Verification items for the finished model (mm, model axes). Face numbers are marked on the shaded views. Give positions to 0.01 mm unless a question says otherwise; leave off trailing zeros. Order: outer loops, then holes, each group sorted by start corner. A loop starts at its lowest first (then second) coordinate and runs counter-clockwise, first axis right, second up.
(1) Sectioned sample at D-D on z = 15. Record the cut outline in (x, y).
(2) Scan lines: L1, parallel to Z at x = 0, y = 0.45; L2, parallel to Z at x = 0, y = 2.15; L3, parallel to Y at x = -25, z = -4.5. Record each from-to range of solid material in increasing order.
(3) Sectioned sample at B-B on z = 0. Record the cut outline in (x, y), plus the area to 3 significant figures.
(4) Sectioned sample at A-A on x = 0. Record the cut outline in (y, z).
(5) Mould release check, pull along Z, two halves, no side actions. Record for the marked faces 1, 2 and 3: pulls with the +Z half, pulls with the -Z half, needs draft (parallel to the pull), parting line crosses it, or undercut.
(6) Sectioned sample at C-C on y = 19. Record the cut outline in (x, z).
(7) Gauge pin test, flat ends, axial feed: pin 1 (10 mm diameter, centred on y = 16, z = 23.5, fed in from +X); pin 2 (4 mm diameter, centred on y = 19, z = 13.5, fed in from -X); pin 3 (1 mm diameter, centred on y = 4.5, z = 27.5, fed in from -X). Record the tip position at first contact, or that the pin passes through.
Autodesk Inventor part; units mm, degrees
ref_plane "YZ Plane" through (0, 0, 0) normal (1, 0, 0) x (0, 1, 0)
ref_plane "XZ Plane" through (0, 0, 0) normal (0, 1, 0) x (-1, 0, 0)
ref_plane "XY Plane" through (0, 0, 0) normal (0, 0, 1) x (1, 0, 0)
sketch "Sketch1" plane through (0, 0, 0) normal (0, 1, 0) x (-1, 0, 0)
  circle A0 centre (0, 0) radius 44
  dimension "d0" = 88
extrude "Extrusion1" add sketch "Sketch1" along normal blind 25
sketch "Sketch2" plane through (0, 25, 0) normal (0, 1, 0) x (1, 0, 0)
  circle A0 centre (0, 0) radius 44
  circle A1 centre (0, 0) radius 39
  dimension "d5" = 5
extrude "Extrusion2" cut sketch "Sketch2" against normal blind 20 contours A1
sketch "Sketch3" plane through (0, 0, 0) normal (0, -1, 0) x (1, 0, 0)
  circle A0 centre (0, 0) radius 3
  circle A1 centre (0, 0) radius 5
  dimension "d8" = 6
  dimension "d9" = 2
extrude "Extrusion3" cut sketch "Sketch3" against normal blind 20 contours A0
extrude "Extrusion4" cut sketch "Sketch3" against normal blind 0.5
fillet "Fillet1" radius 0.2 1 edges at (-5, 0, 0)
sketch "Sketch4" plane through (0, 5, 0) normal (0, 1, 0) x (1, 0, 0)
  circle A0 centre (0, 0) radius 3
  circle A1 centre (0, 0) radius 10
  dimension "d15" = 20
extrude "Extrusion5" cut sketch "Sketch4" against normal blind 0.5
properties part number "bottom" material "Polyethylene, High Density"
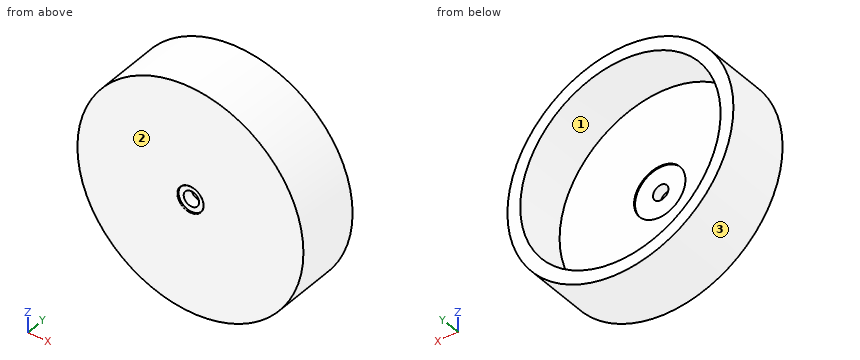
Ans:
1. outline: (-41.36, 0) - (41.36, 0) - (41.36, 25) - (36, 25) - (36, 5) - (-36, 5) - (-36, 25) - (-41.36, 25) - close
2. L1: z = -44 to -5, 5 to 44
2. L2: z = -44 to -3, 3 to 44
2. L3: y = 0 to 5
3. outline: (-44, 0) - (-5.2, 0) arc R0.2 ccw to (-5, 0.2) - (-5, 0.5) - (-3, 0.5) - (-3, 4.5) - (-10, 4.5) - (-10, 5) - (-39, 5) - (-39, 25) - (-44, 25) - close; (3, 0.5) - (5, 0.5) - (5, 0.2) arc R0.2 ccw to (5.2, 0) - (44, 0) - (44, 25) - (39, 25) - (39, 5) - (10, 5) - (10, 4.5) - (3, 4.5) - close
3. area: 601 mm2
4. outline: (0, -44) - (25, -44) - (25, -39) - (5, -39) - (5, -10) - (4.5, -10) - (4.5, -3) - (0.5, -3) - (0.5, -5) - (0.2, -5) arc R0.2 ccw to (0, -5.2) - close; (0, 5.2) arc R0.2 ccw to (0.2, 5) - (0.5, 5) - (0.5, 3) - (4.5, 3) - (4.5, 10) - (5, 10) - (5, 39) - (25, 39) - (25, 44) - (0, 44) - close
5. face 1: undercut
5. face 2: needs draft
5. face 3: parting line crosses it
6. outline: circle Ø88 at (0, 0); hole circle Ø78 at (0, 0)
7. pin 1: stops at x = 39.92
7. pin 2: stops at x = -42.47
7. pin 3: stops at x = -34.74
